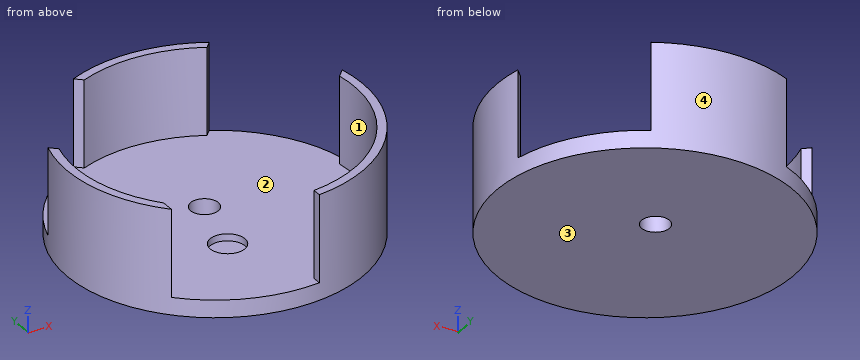
Autodesk Inventor part; units mm, degrees
ref_plane "YZ Plane" through (0, 0, 0) normal (1, 0, 0) x (0, 1, 0)
ref_plane "XZ Plane" through (0, 0, 0) normal (0, 1, 0) x (-1, 0, 0)
ref_plane "XY Plane" through (0, 0, 0) normal (0, 0, 1) x (1, 0, 0)
sketch "Sketch1" plane through (0, 0, 0) normal (0, 0, 1) x (1, 0, 0)
  circle A0 centre (-0.0206, -3.7368) radius 40
  circle A1 centre (-0.0206, -3.7368) radius 42.5
  circle A2 centre (-0.0206, 1.2632) radius 4
  line L0 (-6.0206, 0.0132) -> (5.9794, 0.0132)
  line L1 (5.9794, 0.0132) -> (5.9794, 2.5132)
  line L2 (5.9794, 2.5132) -> (-6.0206, 2.5132)
  line L3 (-6.0206, 2.5132) -> (-6.0206, 0.0132)
  line L4 (-17.3849, 35.0541) -> (-15.3788, 33.1973)
  line L5 (-40.6108, 8.8603) -> (-38.5626, 6.9645)
  line L6 (19.021, 31.4401) -> (21.6473, 34.2375)
  line L7 (39.5419, 2.1626) -> (44.5969, 7.547)
  line L8 (4.4794, -43.4829) -> (4.4794, -45.9979)
  line L9 (-30.5206, -29.6164) -> (-30.5206, -33.3341)
  point P0 (0, 0)
  point P1 (-0.0206, -53.7368)
  point P2 (-0.0206, -9.5426)
  point P3 (-3.8203, 2.5132)
  point P4 (3.779, 2.5132)
  point P5 (3.779, 0.0132)
  point P6 (-3.8203, 0.0132)
  point P7 (-30.452, -29.697)
  point P8 (20.787, 33.3211)
  point P9 (41.6844, 4.4447)
  point P10 (-30.5206, -31.4752)
  dimension "d4" = 40
  dimension "d7" = 50
  dimension "d9" = 8
  dimension "d10" = 12
  dimension "d11" = 2.5
  dimension "d12" = 55
  dimension "d13" = 1.25
  dimension "d14" = 85
  dimension "d15" = 2.5
  dimension "d49" = 35
  dimension "d67" = 35
  dimension "d80" = 35
extrude "Extrusion1" add sketch "Sketch1" along normal blind 5 contours A0 | A0 L7 A1 L8 | A0 L6 A1 L7 | L8 A1 L9 A0 | A0 L4 A1 L6 | L9 A1 L5 A0 | A0 L5 A1 L4 | A2 L0 L2 | A2 L2 L1 L0 | L2 A2 | A2 L0 | A2 L0 L3 L2
extrude "Extrusion10" add sketch "Sketch1" along normal blind 30 contours A0 L7 A1 L8 | A0 L4 A1 L6 | L9 A1 L5 A0 | A2 L0 L2 | L2 A2 | A2 L0
extrude "Extrusion11" cut sketch "Sketch1" along normal blind 30 contours A2 L0 L2 | L2 A2 | A2 L0
sketch "Sketch2" plane through (0, 0, 5) normal (0, 0, 1) x (1, 0, 0)
  circle A0 centre (-0.0206, -3.7368) radius 42.5
  circle A1 centre (-4.787, -17.567) radius 5
  point P0 (0, 0)
  dimension "d94" = 10
extrude "Extrusion12" cut sketch "Sketch2" against normal blind 2 contours A1
properties part number "tryy2"
Source: CAD feature listing. Evaluate the final solid. Frame: model axes, mm. Face numbers are marked on the shaded views. Round coordinates to 2 decimals unless told otherwise and drop trailing zeros. Loops run counter-clockwise (first coordinate to the right, second up) from the corner with the lowest first, then second, coordinate; pieces in that order, holes last. Notation, with made-up numbers: (37, 57) - (94, 57) arc R19 ccw to (94, 66) - close; hole circle Ø5 at (31.25, 69). An arc over 180 degrees is marked (long way). Write item = value, one per line. Start each with the question number.
Item 1: Mould query, pull axis Y, two halves, no side actions, for the marked faces 1, 2, 3 and 4. Classes: released by +Y, released by -Y, zero draft, split by the parting line, or undercut.
Item 2: First-contact query: pin 1 Ø16 at (x, y) = (-4.787, -17.567) entering from -Z; pin 2 Ø6 at (y, z) = (-14.5, 26) entering from +X; pin 3 Ø11 at (x, y) = (-6, -17) entering from +Z; pin 4 Ø4 at (x, z) = (-13, 23) entering from +Y. Flat tips, straight axial feed; report the tip coordinate or a pass-through.
Item 3: Section query A-A on z = 23.5. Output: boundary loops of the cut face in (x, y), plus the area to 3 significant figures.
Item 4: Material intervals for line 1 (Z direction, x = 9, y = -23.5); line 2 (X direction, y = -19.5, z = 11); line 3 (Y direction, x = 14.5, z = 23), sorted ascending.
Item 5: Section query C-C on x = -13. Output: boundary loops of the cut face in (y, z).
Item 6: Section query D-D on y = 18.5. Output: boundary loops of the cut face in (x, z).
Item 7: Section query B-B on x = -2.5. Output: boundary loops of the cut face in (y, z).
Results list:
q1.face_1 = undercut
q1.face_2 = undercut
q1.face_3 = zero draft
q1.face_4 = split by the parting line
q2.pin_1 = 0
q2.pin_2 = 41.76
q2.pin_3 = 5
q2.pin_4 = 37.32
q3.outline = (-40.61, 8.86) arc R42.5 ccw to (-30.52, -33.33) - (-30.52, -29.62) arc R40 cw to (-38.56, 6.96) - close; (-17.38, 35.05) - (-15.38, 33.2) arc R40 cw to (19.02, 31.44) - (20.79, 33.32) arc R42.5 ccw to start; (4.48, -46) arc R42.5 ccw to (41.68, 4.44) - (39.54, 2.16) arc R40 cw to (4.48, -43.48) - close
q3.area = 368 mm²
q4.line_1 = 0 to 5
q4.line_2 = -39.49 to -36.78, 36.74 to 39.45
q4.line_3 = -43.68 to -41.01, 33.53 to 36.21
q5.outline = (-44.21, 0) - (36.73, 0) - (36.73, 30) - (34.1, 30) - (34.1, 5) - (-44.21, 5) - close
q6.outline = (-36.24, 0) - (36.2, 0) - (36.2, 5) - (-36.24, 5) - close
q7.outline = (-46.16, 0) - (-1.88, 0) - (-1.88, 5) - (-13.12, 5) - (-13.12, 3) - (-22.01, 3) - (-22.01, 5) - (-46.16, 5) - close; (4.4, 0) - (38.69, 0) - (38.69, 30) - (36.19, 30) - (36.19, 5) - (4.4, 5) - close
